Answer from the drawing. Dimensions are ordinates in mm from the lowest x, y and z of the part. A direction names the side the tool comes from. Round coordinates to 2 decimals unless told otherwise and drop trailing zeros. Write each loop counter-clockwise with the first axis right and the second up, starting at its lowest first coordinate (ties: lowest second). Pieces come first, ordered by that corner, then holes.
1. A tool of negligible diameter and unlimited length cuts with its end or side. For the marked faces 5, 6 and 7, from which of +Z, -Z, +X, -X, +Y, -Y can it reach the whole face along a straight path? Write none if from no direction.
2. Straight lines are drawn through the part: probe 1 along X at (y, z) = (60.5, 4.5) (1 decimal); probe 2 along X at (y, z) = (40.5, 4.5); probe 3 along Z at (x, y) = (73.5, 52). For each, find the intervals that lie inside material, in ascending order.
3. Find section C-C (y = 12). Write down the section's boundary in (x, z) (1 decimal).
4. Determine the mould class of the marked faces 1, 2, 3 and 4 for opening direction X: pulls with the +X half, pulls with the -X half, needs draft (parallel to the pull), parting line crosses it, or undercut.
5. Flat-ended cylindrical pins translate along their axes: pin 1 Ø5 at (x, z) = (26, 6) entering from +Y; pin 2 Ø2 at (y, z) = (46, 19.5) entering from -X; pin 3 Ø9.5 at (x, z) = (33, 5) entering from -Y; pin 4 Ø7 at (x, y) = (8.5, 6) entering from -Z. Find the tip coordinate at first contact, or state that the pin passes through.
6. Find section A-A (y = 63.5). Count the separate pieces of the cut face and the enclosed holes in it.
7. Find section B-B (x = 5.5). Write down the section's boundary in (y, z) (1 decimal), and give its area (3 significant figures).
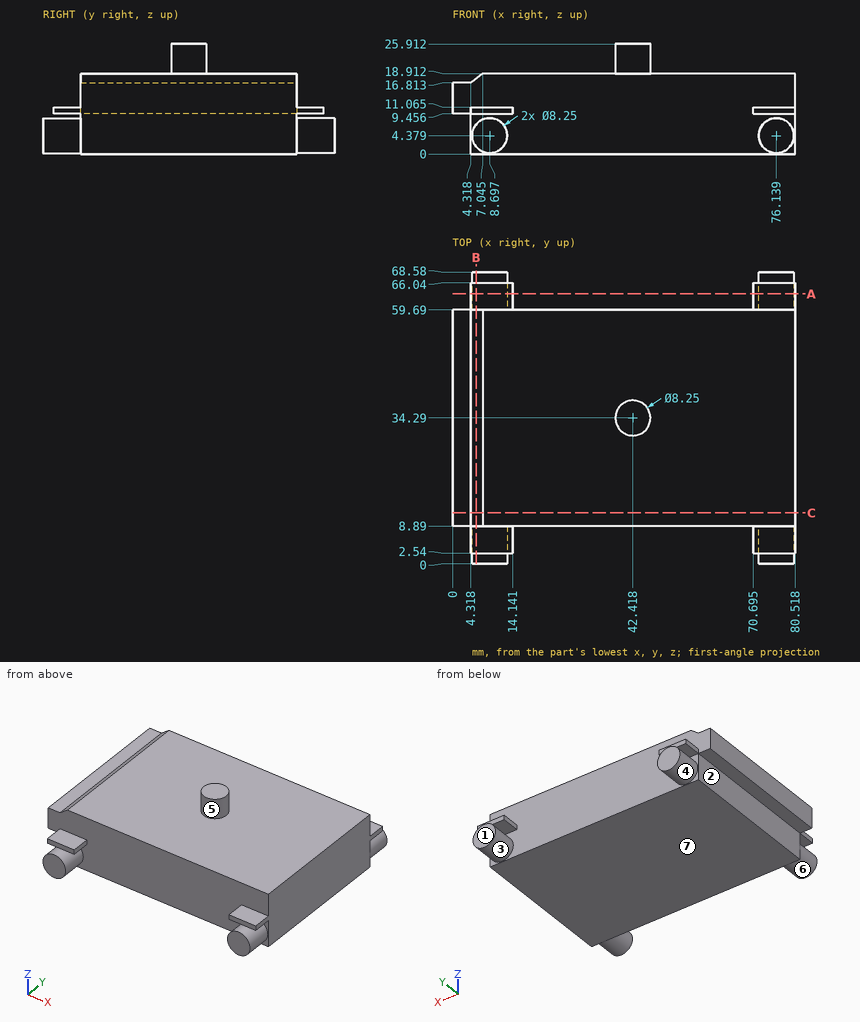
Worked answers:
1. face 5: +Z
1. face 6: -Y
1. face 7: -Z, +X, -X, +Y, -Y
2. probe 1: x = 4.6 to 12.8, 72 to 80.3
2. probe 2: x = 4.32 to 80.52
2. probe 3: z = 0 to 18.91
3. outline: (0, 9.5) - (4.3, 9.5) - (4.3, 0) - (80.5, 0) - (80.5, 18.9) - (7, 18.9) - (4.3, 16.8) - (0, 16.8) - close
4. face 1: needs draft
4. face 2: pulls with the -X half
4. face 3: undercut
4. face 4: undercut
5. pin 1: stops at y = 59.69
5. pin 2: stops at x = 6.51
5. pin 3: stops at y = 8.89
5. pin 4: stops at z = 0
6. separate pieces: 4
6. enclosed holes: 0
7. outline: (0, 1.8) - (8.9, 1.8) - (8.9, 0) - (59.7, 0) - (59.7, 1.8) - (68.6, 1.8) - (68.6, 7) - (59.7, 7) - (59.7, 9.5) - (66, 9.5) - (66, 11.1) - (59.7, 11.1) - (59.7, 17.7) - (8.9, 17.7) - (8.9, 11.1) - (2.5, 11.1) - (2.5, 9.5) - (8.9, 9.5) - (8.9, 7) - (0, 7) - close
7. area: 1,010 mm2
